For this review, take the finished solid that the model builds, in its own axes (mm). Round coordinates to 2 decimals unless told otherwise and drop trailing zeros. Write each loop counter-clockwise with the first axis right and the second up, starting at its lowest first coordinate (ties: lowest second). Pieces come first, ordered by that corner, then holes. Notation, with made-up numbers: (19.25, 76) - (72.25, 76) arc R31 ccw to (72.25, 114) - close; hole circle Ø7 at (28.25, -17). An arc over 180 degrees is marked (long way). One line per item, written item: value. Start each with the question number.
Q1. Clearance check with flat-ended pins moving along their axes: pin 1 Ø5 at (x, z) = (7, 224.5) entering from +Y; pin 2 Ø4 at (x, z) = (-11.5, 164) entering from +Y (3 decimals); pin 3 Ø8 at (y, z) = (48, 193.5) entering from -X; pin 4 Ø6 at (y, z) = (-3, 105) entering from +X. State where each tip first meets the part, or that it passes through.
Q2. Add section A-A on z = 93.5. Write out the cut boundary in (x, y).
Q3. Add section B-B on z = 10. Write out the cut boundary in (x, y).
Q4. Mouldability with a two-part tool opening along X and no side actions: class faces 1 (the face through (0, 0, 320)), 2 (the face through (18.811, -14.423, 287.111)), 3 (the face through (59.54, 42.91, 13)) as +X half, -X half, draft (parallel to the pull), parting line (faces both ways), or undercut.
Q5. For probe 1 along X at (y, z) = (2, 44.5); probe 2 along Z at (x, y) = (24, 2); probe 3 along X at (y, z) = (31.5, 59.5), list the stretches that pass through material, from the lowest coordinate up.
Autodesk Fusion 360 part; units mm, degrees
sketch "Sketch1" plane through (0, 0, 0) normal (0, 0, 1) x (1, 0, 0)
  circle A0 centre (0, 0) radius 60
  dimension "d1" = 120
extrude "Extrude1" add sketch "Sketch1" along normal blind 200
sketch "Sketch2" plane through (0, 0, 0) normal (0, 1, 0) x (1, 0, 0)
  line L0 (70, -110) -> (70, -115.5379)
  line L1 (-60, -200) -> (-10, -320)
  line L2 (-10, -320) -> (0, -320)
  line L3 (0, -320) -> (0, -200)
  line L4 (0, -200) -> (-60, -200)
revolve "Revolve1" add sketch "Sketch2" angle 360 about axis through (0, 0, 320) along (0, 0, -1)
fillet "Fillet1" radius 200 1 edges at (-55.9396, -21.6969, 200)
sketch "Sketch4" plane through (0, 0, 0) normal (0, 1, 0) x (1, 0, 0)
  circle A0 centre (50, -10) radius 10
extrude "Extrude2" add sketch "Sketch4" along normal blind 60
Result set:
1. pin 1: stops at y = 49.72
1. pin 2: stops at y = 59.205
1. pin 3: stops at x = -36.62
1. pin 4: stops at x = 60
2. outline: circle Ø120 at (0, 0)
3. outline: (40, 44.72) arc R60 ccw (long way) to (60, 0) - (60, 60) - (40, 60) - close
4. face 1: draft
4. face 2: parting line
4. face 3: undercut
5. probe 1: x = -59.97 to 59.97
5. probe 2: z = 0 to 286.2
5. probe 3: x = -51.07 to 51.07
